```python
from build123d import *

# Parameters (mm, degrees)
SKETCH1_W          = 40
SKETCH1_H          = 20
MAIN_BODY_DEPTH    = 30
SKETCH2_W          = 50
SKETCH2_H          = 30
FLANGE_1_DEPTH     = 2.5
SKETCH4_W          = 50
SKETCH4_H          = 30
SKETCH4_W_2        = 40
SKETCH4_H_2        = 20
FLANGE_2_DEPTH     = 2.5
SKETCH5_R          = 5
HOLE_DEPTH         = 46.552167896
MAIN_BODY_FILLET_R = 2
FLANGE_FILLET_R    = 1


with BuildPart() as part:
    # Sketch1 → Main Body (new body)
    with BuildSketch(Plane(origin=(0, 0, 0), x_dir=(1, 0, 0), z_dir=(0, 1, 0))):
        Rectangle(SKETCH1_W, SKETCH1_H)
    extrude(amount=MAIN_BODY_DEPTH)

    # Sketch2 → Flange 1 (add)
    with BuildSketch(Plane(origin=(0, 30, 0), x_dir=(1, 0, 0), z_dir=(0, 1, 0))):
        Rectangle(SKETCH2_W, SKETCH2_H)
    extrude(amount=FLANGE_1_DEPTH)

    # Sketch4 → Flange 2 (add)
    # profile 1 of 2: a face of its own
    with BuildSketch(Plane.XZ):
        Rectangle(SKETCH4_W, SKETCH4_H)
        Rectangle(SKETCH4_W_2, SKETCH4_H_2, mode=Mode.SUBTRACT)
    # profile 2 of 2: a face of its own
    with BuildSketch(Plane.XZ):
        Rectangle(SKETCH4_W_2, SKETCH4_H_2)
    extrude(amount=FLANGE_2_DEPTH)

    # Sketch5 → Hole (cut, through all)
    with BuildSketch(Plane(origin=(0, 32.5, 0), x_dir=(1, 0, 0), z_dir=(0, 1, 0))):
        with Locations(Location((0, 0, 0), (0, 0, 270))):
            Circle(SKETCH5_R)
    extrude(amount=-HOLE_DEPTH, mode=Mode.SUBTRACT)

    # Main Body Fillet
    main_body_fillet_edges = [part.edges().sort_by_distance(p)[0] for p in [
        (20, 15, 10),
        (-20, 15, 10),
        (-20, 15, -10),
        (20, 15, -10),
    ]]
    fillet(main_body_fillet_edges, radius=MAIN_BODY_FILLET_R)

    # Flange Fillet
    flange_fillet_edges = [part.edges().sort_by_distance(p)[0] for p in [
        (25, 31.25, 15),
        (25, 31.25, -15),
        (-25, 31.25, -15),
        (-25, 31.25, 15),
        (25, -1.25, 15),
        (-25, -1.25, 15),
        (-25, -1.25, -15),
        (25, -1.25, -15),
    ]]
    fillet(flange_fillet_edges, radius=FLANGE_FILLET_R)


solid = part.part
```
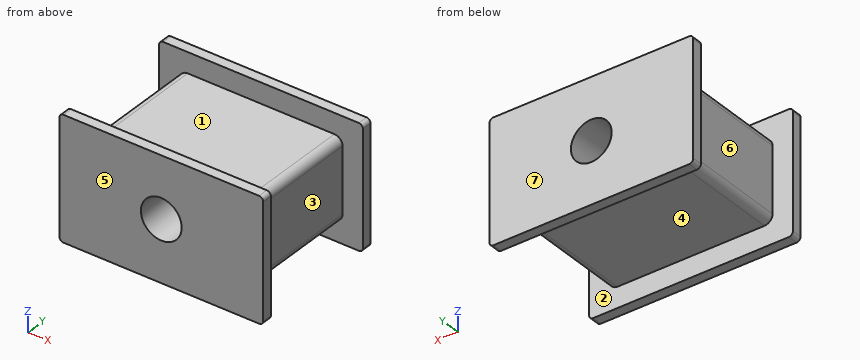
Check sheet for the modelled part. Datum: model origin and axes. Units: mm. Face numbers are marked on the shaded views. A direction names the side the tool comes from. Round coordinates to 2 decimals unless told otherwise and drop trailing zeros. Loops run counter-clockwise (first coordinate to the right, second up) from the corner with the lowest first, then second, coordinate; pieces in that order, holes last. Notation, with made-up numbers: (-28.75, 4) -> (5.25, 4) arc R34 cw to (5.25, 42) -> close; hole circle Ø2 at (80.5, 47). An arc over 180 degrees is marked (long way). Answer in a Markdown table with one row per item.
Q1. Set-up check for the marked faces 1, 2, 3 and 4: record each of +Z, -Z, +X, -X, +Y, -Y from which the full face is reachable in a straight line by a thin tool's end or side.
Data:
| item | result |
|---|---|
| face 1 | +Z, +X, -X |
| face 2 | none |
| face 3 | +Z, -Z, +X |
| face 4 | -Z, +X, -X |
Q2. Sectioned sample at A-A on x = 0. Enter the section's corners in (y, z).
Data:
| item | result |
|---|---|
| outline | (-2.5, -15) -> (0, -15) -> (0, -10) -> (30, -10) -> (30, -15) -> (32.5, -15) -> (32.5, -5) -> (-2.5, -5) -> close; (-2.5, 5) -> (32.5, 5) -> (32.5, 15) -> (30, 15) -> (30, 10) -> (0, 10) -> (0, 15) -> (-2.5, 15) -> close |
Q3. Sectioned sample at B-B on z = -4. Enter the section's corners in (x, y), then the cut area to 3 significant figures.
Data:
| item | result |
|---|---|
| outline | (-25, -2.5) -> (-3, -2.5) -> (-3, 32.5) -> (-25, 32.5) -> (-25, 30) -> (-20, 30) -> (-20, 0) -> (-25, 0) -> close; (3, -2.5) -> (25, -2.5) -> (25, 0) -> (20, 0) -> (20, 30) -> (25, 30) -> (25, 32.5) -> (3, 32.5) -> close |
| area | 1,240 mm^2 |
Q4. Thickness scan on L1, parallel to X at y = 11, z = 0; L2, parallel to Z at x = -13, y = 29.5; L3, parallel to Y at x = -6.5, z = 10.5. Record the ranges inside material, lowest first.
Data:
| item | result |
|---|---|
| L1 | x = -20 to -5, 5 to 20 |
| L2 | z = -10 to 10 |
| L3 | y = -2.5 to 0, 30 to 32.5 |
Q5. Sectioned sample at D-D on z = -7.25. Enter the section's corners in (x, y), then the cut area to 3 significant figures.
Data:
| item | result |
|---|---|
| outline | (-25, -2.5) -> (25, -2.5) -> (25, 0) -> (20, 0) -> (20, 30) -> (25, 30) -> (25, 32.5) -> (-25, 32.5) -> (-25, 30) -> (-20, 30) -> (-20, 0) -> (-25, 0) -> close |
| area | 1,450 mm^2 |
Q6. Release check for a two-part mould opening along Y. For the marked faces 5, 6 and 7 record: released by +Y, released by -Y, zero draft, split by the parting line, or undercut.
Data:
| item | result |
|---|---|
| face 5 | released by -Y |
| face 6 | undercut |
| face 7 | released by +Y |
Q7. Go/stop test with flat-tipped pins: P1, Ø9, axis at x = -6.5, y = 14, coming from the -Z side; P2, Ø10, axis at y = 24, z = 6.5, coming from the +X side; P3, Ø15, axis at x = 3.5, y = 9, coming from the +Z side. Record where each tip stops, or that it passes through.
Data:
| item | result |
|---|---|
| P1 | stops at z = -10 |
| P2 | stops at x = 20 |
| P3 | stops at z = 10 |
Q8. Sectioned sample at C-C on y = 17.5. Enter the section's corners in (x, z), then the cut area to 3 significant figures.
Data:
| item | result |
|---|---|
| outline | (-20, -8) arc R2 ccw to (-18, -10) -> (18, -10) arc R2 ccw to (20, -8) -> (20, 8) arc R2 ccw to (18, 10) -> (-18, 10) arc R2 ccw to (-20, 8) -> close; hole circle Ø10 at (0, 0) |
| area | 718 mm^2 |
